The model under review builds one solid part; all positions refer to its coordinate system, in mm. A direction names the side the tool comes from. Coordinates: 2 decimals unless noted, no trailing zeros. Order: outer loops, then holes, each group sorted by start corner. A loop starts at its lowest first (then second) coordinate and runs counter-clockwise, first axis right, second up. Notation, with made-up numbers: (-26.75, -26.5) -> (13.25, -26.5) arc R19 ccw to (13.25, -20.5) -> close; hole circle Ø1 at (6.25, -38). An arc over 180 degrees is marked (long way). Put each result on its own line as item: value.
from build123d import *

# Parameters (mm, degrees)
F0_W      = 152.4
F0_H      = 115.57
F1_DEPTH  = 19.05
F3_DEPTH  = 5.08
F4_W      = 114.3
F4_H      = 6.35
F5_DEPTH  = 7.112
F6_DEPTH  = 0.79375
F7_W      = 152.4
F7_H      = 5.715
F8_DEPTH  = 17.4625
F9_DEPTH  = 1.27
F10_R     = 6.35
F11_DEPTH = 9.525
F12_R     = 4.45
F12_R_2   = 4.445
F13_DEPTH = 10.16


with BuildPart() as f1:
    # F0 (on Top) → F1 (new body)
    with BuildSketch(Plane.XY):
        with Locations((76.2, 57.785)):
            Rectangle(F0_W, F0_H)
    extrude(amount=F1_DEPTH)

    # F2 (on face) → F3 (cut)
    with BuildSketch(Plane.XY.offset(19.05)):
        with BuildLine():
            Line((140.335, 113.03), (12.065, 113.03))
            ThreePointArc((12.065, 113.03), (5.329808, 110.240192), (2.54, 103.505))
            Line((2.54, 103.505), (2.54, 12.065))
            ThreePointArc((2.54, 12.065), (5.329808, 5.329808), (12.065, 2.54))
            Line((12.065, 2.54), (140.335, 2.54))
            ThreePointArc((140.335, 2.54), (147.070192, 5.329808), (149.86, 12.065))
            Line((149.86, 12.065), (149.86, 103.505))
            ThreePointArc((149.86, 103.505), (147.070192, 110.240192), (140.335, 113.03))
        make_face()
        with BuildLine():
            ThreePointArc((8.89, 103.505), (9.819936, 105.750064), (12.065, 106.68))
            Line((12.065, 106.68), (140.335, 106.68))
            ThreePointArc((140.335, 106.68), (142.580064, 105.750064), (143.51, 103.505))
            Line((143.51, 103.505), (143.51, 12.065))
            ThreePointArc((143.51, 12.065), (142.580064, 9.819936), (140.335, 8.89))
            Line((140.335, 8.89), (12.065, 8.89))
            ThreePointArc((12.065, 8.89), (9.819936, 9.819936), (8.89, 12.065))
            Line((8.89, 12.065), (8.89, 103.505))
        make_face(mode=Mode.SUBTRACT)
    extrude(amount=-F3_DEPTH, mode=Mode.SUBTRACT)

    # F4 (on face) → F5 (cut)
    with BuildSketch(Plane.XY.offset(19.05)):
        with Locations((76.2, 57.785)):
            Rectangle(F4_W, F4_H)
        with Locations((76.2, 79.785)):
            Rectangle(F4_W, F4_H)
        with Locations((76.2, 35.785)):
            Rectangle(F4_W, F4_H)
    extrude(amount=-F5_DEPTH, mode=Mode.SUBTRACT)

    # F2 (on face) → F6 (cut)
    with BuildSketch(Plane.XY.offset(19.05)):
        with BuildLine():
            Line((140.335, 106.68), (12.065, 106.68))
            ThreePointArc((12.065, 106.68), (9.819936, 105.750064), (8.89, 103.505))
            Line((8.89, 103.505), (8.89, 12.065))
            ThreePointArc((8.89, 12.065), (9.819936, 9.819936), (12.065, 8.89))
            Line((12.065, 8.89), (140.335, 8.89))
            ThreePointArc((140.335, 8.89), (142.580064, 9.819936), (143.51, 12.065))
            Line((143.51, 12.065), (143.51, 103.505))
            ThreePointArc((143.51, 103.505), (142.580064, 105.750064), (140.335, 106.68))
        make_face()
    extrude(amount=-F6_DEPTH, mode=Mode.SUBTRACT)

    # F7 (on face) → F8 (join)
    with BuildSketch(Plane.XY):
        with Locations((76.2, -2.8575)):
            Rectangle(F7_W, F7_H)
        with Locations((76.2, 118.4275)):
            Rectangle(F7_W, F7_H)
    extrude(amount=F8_DEPTH)

    # F2 (on face) → F9 (cut)
    with BuildSketch(Plane.XY.offset(19.05)):
        with BuildLine():
            Line((140.335, 106.68), (12.065, 106.68))
            ThreePointArc((12.065, 106.68), (9.819936, 105.750064), (8.89, 103.505))
            Line((8.89, 103.505), (8.89, 12.065))
            ThreePointArc((8.89, 12.065), (9.819936, 9.819936), (12.065, 8.89))
            Line((12.065, 8.89), (140.335, 8.89))
            ThreePointArc((140.335, 8.89), (142.580064, 9.819936), (143.51, 12.065))
            Line((143.51, 12.065), (143.51, 103.505))
            ThreePointArc((143.51, 103.505), (142.580064, 105.750064), (140.335, 106.68))
        make_face()
    extrude(amount=-F9_DEPTH, mode=Mode.SUBTRACT)

    # F10 (on face) → F11 (cut)
    with BuildSketch(Plane.XY.offset(19.05)):
        with Locations((16.51, 99.06)):
            Circle(F10_R)
        with Locations((135.89, 99.06)):
            Circle(F10_R)
        with Locations((16.51, 16.51)):
            Circle(F10_R)
        with Locations((135.89, 16.51)):
            Circle(F10_R)
    extrude(amount=-F11_DEPTH, mode=Mode.SUBTRACT)

    # F12 (on face) → F13 (cut)
    with BuildSketch(Plane.XY):
        with Locations((76.2, 57.785)):
            Circle(F12_R)
        with Locations((44.45, 57.785)):
            Circle(F12_R_2)
        with Locations((53.74936, 35.33436)):
            Circle(F12_R_2)
        with Locations((76.2, 26.035)):
            Circle(F12_R_2)
        with Locations((98.65064, 35.33436)):
            Circle(F12_R_2)
        with Locations((107.95, 57.785)):
            Circle(F12_R_2)
        with Locations((98.65064, 80.23564)):
            Circle(F12_R_2)
        with Locations((76.2, 89.535)):
            Circle(F12_R_2)
        with Locations((53.74936, 80.23564)):
            Circle(F12_R_2)
    extrude(amount=F13_DEPTH, mode=Mode.SUBTRACT)


solid = f1.part
Item 1: Consider section D-D on y = 42. Write out the cut boundary in (x, z).
Answers below:
outline: (0, 0) -> (152.4, 0) -> (152.4, 19.05) -> (149.86, 19.05) -> (149.86, 13.97) -> (143.51, 13.97) -> (143.51, 17.78) -> (8.89, 17.78) -> (8.89, 13.97) -> (2.54, 13.97) -> (2.54, 19.05) -> (0, 19.05) -> close
Item 2: Consider section B-B on z = 3.75. Count the separate pieces of the cut face and the enclosed holes in it, and give its area (3 significant figures).
Answers below:
separate pieces: 1
enclosed holes: 9
area: 18,800 mm^2
Item 3: Consider section A-A on y = 16.51. Write out the cut boundary in (x, z) (3 decimals), and give its area (3 significant figures).
Answers below:
outline: (0, 0) -> (152.4, 0) -> (152.4, 19.05) -> (149.86, 19.05) -> (149.86, 13.97) -> (143.51, 13.97) -> (143.51, 17.78) -> (142.24, 17.78) -> (142.24, 9.525) -> (129.54, 9.525) -> (129.54, 17.78) -> (22.86, 17.78) -> (22.86, 9.525) -> (10.16, 9.525) -> (10.16, 17.78) -> (8.89, 17.78) -> (8.89, 13.97) -> (2.54, 13.97) -> (2.54, 19.05) -> (0, 19.05) -> close
area: 2,460 mm^2
Item 4: For faces 3 (the flat face through (77, 113.03, 17)), 4 (the cylindrical face through (78.25, 22.09, 5.01)), list the 3-axis set-ups (+Z, -Z, +X, -X, +Y, -Y) from which the entire face can be reached by the end or side of a thin tool; tool diameter is ignored.
Answers below:
face 3: +Z
face 4: -Z
Item 5: Mouldability with a two-part tool opening along X and no side actions: class faces 1 (the flat face through (75, -3, 17.462)), 2 (the flat face through (75, 48, 17.78)) as +X half, -X half, draft (parallel to the pull), parting line (faces both ways), or undercut.
Answers below:
face 1: draft
face 2: undercut
Item 6: For pin 1 Ø11.5 at (x, y) = (16.51, 99.06) entering from +Z (3 decimals); pin 2 Ø3 at (x, y) = (102.5, 50) entering from +Z; pin 3 Ø3 at (x, y) = (81, 78.5) entering from +Z, all flat-tipped, find the tip position at first contact; note any pin that passes through.
Answers below:
pin 1: z = 9.525
pin 2: z = 17.78
pin 3: z = 11.94
Item 7: For line 1 (Y direction, x = 76.2, z = 8.25) (3 decimals); line 2 (Y direction, x = 16.51, z = 11.5) (3 decimals); line 3 (Y direction, x = 80.5, z = 15.5) (3 decimals), list the stretches that pass through material, from the lowest coordinate up. Write a range as from..to.
Answers below:
line 1: -5.715..21.59, 30.48..53.335, 62.235..85.09, 93.98..121.285
line 2: -5.715..10.16, 22.86..92.71, 105.41..121.285
line 3: -5.715..2.54, 8.89..32.61, 38.96..54.61, 60.96..76.61, 82.96..106.68, 113.03..121.285
